Here's how the part is built. I have some questions about the finished solid (model axes, mm). Face numbers are marked on the shaded views. Coordinates: 2 decimals unless noted, no trailing zeros. Write each loop counter-clockwise with the first axis right and the second up, starting at its lowest first coordinate (ties: lowest second). Pieces come first, ordered by that corner, then holes. Notation, with made-up numbers: (85.5, -37) -> (141.5, -37) arc R22 cw to (141.5, -8) -> close; hole circle Ø8 at (73.25, 44.25). An arc over 180 degrees is marked (long way). Use a Markdown table: item, result. Add a question column.
Autodesk Inventor part; units mm, degrees
ref_plane "YZ Plane" through (0, 0, 0) normal (1, 0, 0) x (0, 1, 0)
ref_plane "XZ Plane" through (0, 0, 0) normal (0, 1, 0) x (-1, 0, 0)
ref_plane "XY Plane" through (0, 0, 0) normal (0, 0, 1) x (1, 0, 0)
sketch "Sketch1" plane through (0, 0, 0) normal (0, 0, 1) x (1, 0, 0)
  circle A0 centre (0, 0) radius 9.525
  circle A1 centre (0, 0) radius 25.4 construction
  circle A2 centre (-30.1625, 0) radius 4.7625 construction
  circle A3 centre (30.1625, 0) radius 4.7625 construction
  circle A4 centre (0, 0) radius 17.4625 construction
  line L0 (-17.3789, 18.5238) -> (-33.4211, 3.4732)
  line L1 (-33.4211, -3.4732) -> (-17.3789, -18.5238)
  line L2 (17.3789, -18.5238) -> (33.4211, -3.4732)
  line L3 (33.4211, 3.4732) -> (17.3789, 18.5238)
  arc A5 (-33.4211, 3.4732) -> (-33.4211, -3.4732) centre (-30.1625, 0) ccw
  arc A6 (-17.3789, -18.5238) -> (17.3789, -18.5238) centre (0, 0) ccw
  arc A7 (33.4211, -3.4732) -> (33.4211, 3.4732) centre (30.1625, 0) ccw
  arc A8 (17.3789, 18.5238) -> (-17.3789, 18.5238) centre (0, 0) ccw
  point P0 (-17.4625, 0)
  point P1 (-8.7313, -15.123)
  point P2 (8.7312, -15.123)
  point P3 (17.4625, 0)
  point P4 (8.7313, 15.123)
  point P5 (-8.7312, 15.123)
  dimension "d3" = 34.925
  dimension "d0" = 19.05
  dimension "d1" = 50.8
  dimension "d2" = 9.525
  dimension "d6" = 360
extrude "Extrusion1" add sketch "Sketch1" along normal blind 6.35
hole "Hole1" at (-17.4625, 0, 0) at (-8.7313, -15.123, 0) at (8.7312, -15.123, 0) at (17.4625, 0, 0) at (8.7313, 15.123, 0) at (-8.7312, 15.123, 0) at (-30.1625, 0, 0) at (30.1625, 0, 0) direction (0, 0, 1) diameter 5.1054 end through all
properties part number "GP7-003" material "Polycarbonate, Smoke"
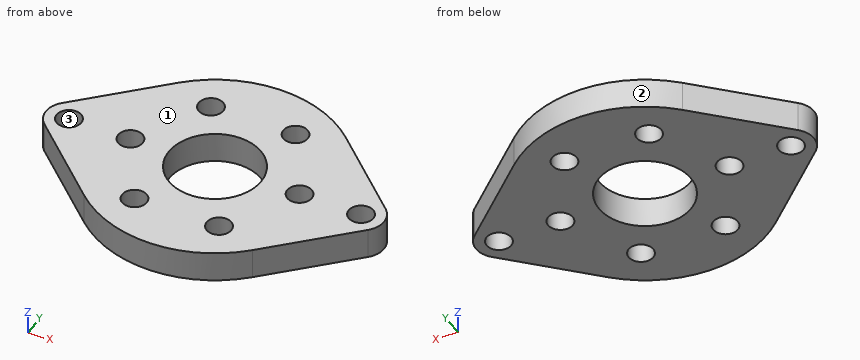
Q1. Please list where these lines run through material, in increasing order: line 1 (Y direction, x = 0, z = 3.5) (3 decimals); line 2 (X direction, y = 1, z = 2.25); line 3 (Y direction, x = 5, z = 1.25).
Q2. Suppose I cut it at D-D, the plane y = 13.5. Write out the boundary of the cut face in (x, z), and give its area (3 significant figures).
Q3. Will these pins go through, and if not, where does the flat tip stop? pin 1 (1 mm diameter, centred on x = 22, z = 2, fed in from -Y); pin 2 (2 mm diameter, centred on x = -4.5, z = 4.5, fed in from -Y).
Q4. Thinking about a two-plate mould opening in X: for the marked faces 1, 2 and 3, which applies, released by +X, released by -X, zero draft, split by the parting line, or undercut?
Q5. Suppose I cut it at C-C, the plane z = 3.5. State how many separate pieces and enclosed holes the cut face has, and give its area (3 significant figures).
Q6. Suppose I cut it at A-A, the plane x = 0. Write out the boundary of the cut face in (y, z) (3 decimals), and give its area (3 significant figures).
Q7. Suppose I cut it at B-B, the plane y = 0. Write out the boundary of the cut face in (x, z) (3 decimals), and give its area (3 significant figures).
Answer key:
| question | item | result |
|---|---|---|
| 1 | line 1 | y = -25.4 to -9.525, 9.525 to 25.4 |
| 1 | line 2 | x = -34.82 to -32.51, -27.81 to -19.81, -15.11 to -9.47, 9.47 to 15.11, 19.81 to 27.81, 32.51 to 34.82 |
| 1 | line 3 | y = -24.9 to -8.11, 8.11 to 24.9 |
| 2 | outline | (-22.73, 0) -> (-10.7, 0) -> (-10.7, 6.35) -> (-22.73, 6.35) -> close; (-6.76, 0) -> (6.76, 0) -> (6.76, 6.35) -> (-6.76, 6.35) -> close; (10.7, 0) -> (22.73, 0) -> (22.73, 6.35) -> (10.7, 6.35) -> close |
| 2 | area | 239 mm^2 |
| 3 | pin 1 | stops at y = -14.66 |
| 3 | pin 2 | stops at y = -25.16 |
| 4 | face 1 | zero draft |
| 4 | face 2 | split by the parting line |
| 4 | face 3 | undercut |
| 5 | separate pieces | 1 |
| 5 | enclosed holes | 9 |
| 5 | area | 1,890 mm^2 |
| 6 | outline | (-25.4, 0) -> (-9.525, 0) -> (-9.525, 6.35) -> (-25.4, 6.35) -> close; (9.525, 0) -> (25.4, 0) -> (25.4, 6.35) -> (9.525, 6.35) -> close |
| 6 | area | 202 mm^2 |
| 7 | outline | (-34.925, 0) -> (-32.715, 0) -> (-32.715, 6.35) -> (-34.925, 6.35) -> close; (-27.61, 0) -> (-20.015, 0) -> (-20.015, 6.35) -> (-27.61, 6.35) -> close; (-14.91, 0) -> (-9.525, 0) -> (-9.525, 6.35) -> (-14.91, 6.35) -> close; (9.525, 0) -> (14.91, 0) -> (14.91, 6.35) -> (9.525, 6.35) -> close; (20.015, 0) -> (27.61, 0) -> (27.61, 6.35) -> (20.015, 6.35) -> close; (32.715, 0) -> (34.925, 0) -> (34.925, 6.35) -> (32.715, 6.35) -> close |
| 7 | area | 193 mm^2 |
